Check sheet for the drawn part. Datum: minimum x, y, z corner. Units: mm. A direction names the side the tool comes from. Give positions to 0.01 mm unless a question says otherwise; leave off trailing zeros. Write each loop counter-clockwise with the first axis right and the second up, starting at its lowest first coordinate (ties: lowest second). Pieces come first, ordered by that corner, then holes. Notation, with made-up numbers: (-22.75, 8.5) - (6.25, 8.5) arc R14 cw to (6.25, 25.5) - close; hole circle Ø5 at (24.25, 44.25). An arc over 180 degrees is marked (long way). One line per question, with ' | ' between items. Start each with the question number.
Q1. Section check B-B on x = 26. Record the boundary of the cut face in (y, z), and give its area (3 significant figures).
Q2. Gauge pin test, flat ends, axial feed: P1, Ø2, axis at y = 11, z = 20.5, coming from the -X side; P2, Ø11, axis at y = 13.5, z = 39, coming from the +X side; P3, Ø5, axis at y = 14.5, z = 41, coming from the -X side; P4, Ø3, axis at x = 27.5, z = 44.5, coming from the -Y side. Record the tip position at first contact, or that the pin passes through.
Q3. Section check D-D on x = 44. Record the boundary of the cut face in (y, z), and give its area (3 significant figures).
Q4. Section check A-A on y = 12.5. Record the boundary of the cut face in (x, z), and give its area (3 significant figures).
Q5. Set-up check for the marked faces 1, 2, 3, 4 and 5: record each of +Z, -Z, +X, -X, +Y, -Y from which the full face is reachable in a straight line by a thin tool's end or side.
Q6. Thickness scan on L1, parallel to Z at x = 18, y = 15.25; L2, parallel to Y at x = 27.5, z = 48; L3, parallel to X at y = 17.75, z = 26.5. Record the ranges inside material, lowest first. Write a range as [from, to].
Q7. Section check C-C on z = 40.5. Record the boundary of the cut face in (x, y), and give its area (3 significant figures).
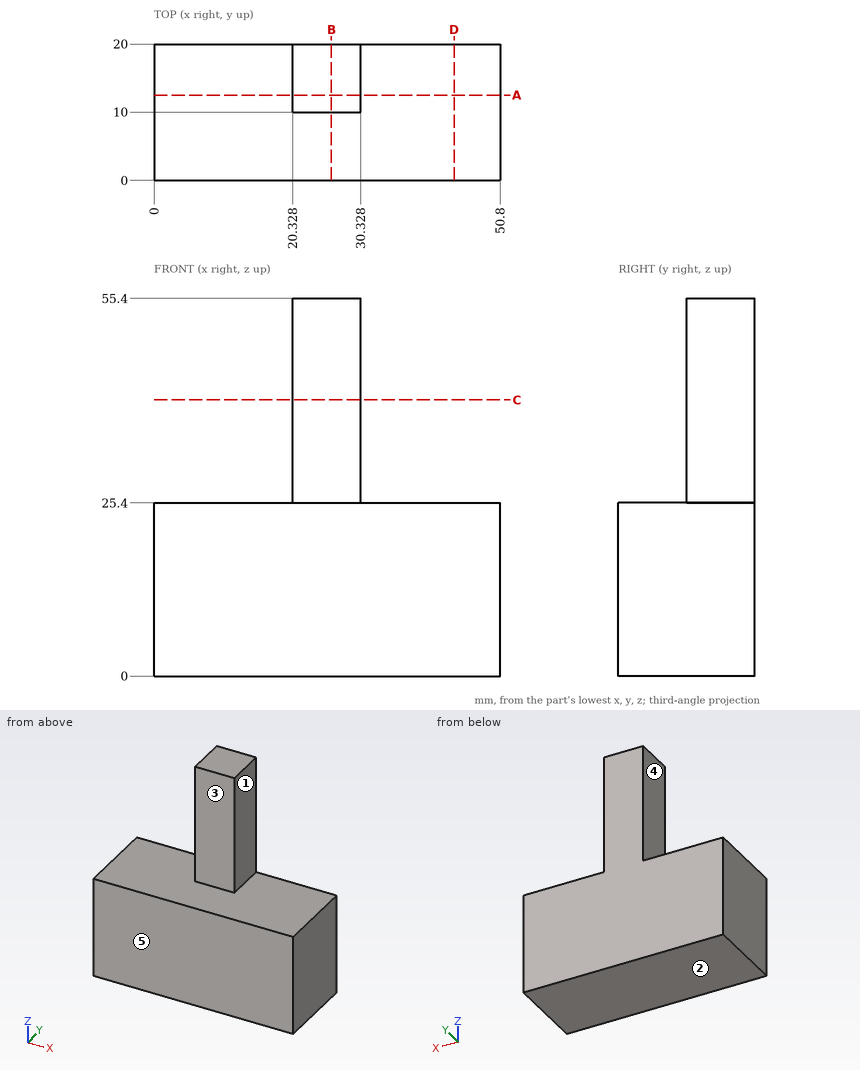
Working result:
1) outline: (0, 0) - (20, 0) - (20, 55.4) - (10, 55.4) - (10, 25.4) - (0, 25.4) - close | area: 808 mm2
2) P1: stops at x = 0 | P2: stops at x = 30.33 | P3: stops at x = 20.33 | P4: stops at y = 10
3) outline: (0, 0) - (20, 0) - (20, 25.4) - (0, 25.4) - close | area: 508 mm2
4) outline: (0, 0) - (50.8, 0) - (50.8, 25.4) - (30.33, 25.4) - (30.33, 55.4) - (20.33, 55.4) - (20.33, 25.4) - (0, 25.4) - close | area: 1,590 mm2
5) face 1: +Z, +X, +Y, -Y | face 2: -Z, +X, -X, +Y, -Y | face 3: +Z, +X, -X, -Y | face 4: +Z, -X, +Y, -Y | face 5: +Z, -Z, +X, -X, -Y
6) L1: z = [0, 25.4] | L2: y = [10, 20] | L3: x = [20.33, 30.33]
7) outline: (20.33, 10) - (30.33, 10) - (30.33, 20) - (20.33, 20) - close | area: 100 mm2
